Source: CAD feature listing. Evaluate the final solid. Frame: model axes, mm. A direction names the side the tool comes from. Coordinates: 2 decimals unless noted, no trailing zeros. Write each loop counter-clockwise with the first axis right and the second up, starting at its lowest first coordinate (ties: lowest second). Pieces come first, ordered by that corner, then holes. Notation, with made-up numbers: (88.25, -1.5) -> (112.25, -1.5) arc R35 cw to (112.25, 30.5) -> close; hole circle Ø11 at (-20.75, -37.5). An arc over 180 degrees is marked (long way). Write item = value, one per line.
from build123d import *

# Parameters (mm, degrees)
SKETCH1_R             = 3
BOSS_EXTRUDE1_DEPTH   = 2
SKETCH1_R_2           = 1.575
SKETCH1_R_3           = 4.75
BOSS_EXTRUDE1_2_DEPTH = 2
BOSS_EXTRUDE2_DEPTH   = 5.2
FILLET1_R             = 1


with BuildPart() as part:
    # Sketch1 → Boss-Extrude1 (new body)
    with BuildSketch(Plane(origin=(0, 0, 0), x_dir=(1, 0, 0), z_dir=(0, 1, 0))):
        with Locations(Location((0, 0, 0), (0, 0, 270))):
            Circle(SKETCH1_R)
    extrude(amount=BOSS_EXTRUDE1_DEPTH)



with BuildPart() as body_2:
    # Sketch1 → Boss-Extrude1 2 (new body)
    with BuildSketch(Plane(origin=(0, 0, 0), x_dir=(1, 0, 0), z_dir=(0, 1, 0))):
        with BuildLine():
            Line((-2.785823381, 7.172375213), (-8.27733707, 15.397108965))
            Line((-8.27733707, 15.397108965), (-15.361972878, 8.339635234))
            Line((-15.361972878, 8.339635234), (-7.163433576, 2.808735927))
            ThreePointArc((-7.163433576, 2.808735927), (-7.694389311, 0.01229774), (-7.172375213, -2.785823381))
            Line((-7.172375213, -2.785823381), (-15.397108965, -8.27733707))
            Line((-15.397108965, -8.27733707), (-8.339635234, -15.361972878))
            Line((-8.339635234, -15.361972878), (-2.808735927, -7.163433576))
            ThreePointArc((-2.808735927, -7.163433576), (-0.01229774, -7.694389311), (2.785823381, -7.172375213))
            Line((2.785823381, -7.172375213), (8.27733707, -15.397108965))
            Line((8.27733707, -15.397108965), (15.361972878, -8.339635234))
            Line((15.361972878, -8.339635234), (7.163433576, -2.808735927))
            ThreePointArc((7.163433576, -2.808735927), (7.694389311, -0.01229774), (7.172375213, 2.785823381))
            Line((7.172375213, 2.785823381), (15.397108965, 8.27733707))
            Line((15.397108965, 8.27733707), (8.339635234, 15.361972878))
            Line((8.339635234, 15.361972878), (2.808735927, 7.163433576))
            ThreePointArc((2.808735927, 7.163433576), (0.01229774, 7.694389311), (-2.785823381, 7.172375213))
        make_face()
        with Locations(Location((7.61701493, 7.585748715, 0), (0, 0, 270))):
            Circle(SKETCH1_R_2, mode=Mode.SUBTRACT)
        with Locations(Location((0, 0, 0), (0, 0, 270))):
            Circle(SKETCH1_R_3, mode=Mode.SUBTRACT)
        with Locations(Location((-7.61701493, -7.585748715, 0), (0, 0, 270))):
            Circle(SKETCH1_R_2, mode=Mode.SUBTRACT)
        with Locations(Location((-7.585748715, 7.61701493, 0), (0, 0, 270))):
            Circle(SKETCH1_R_2, mode=Mode.SUBTRACT)
        with Locations(Location((7.585748715, -7.61701493, 0), (0, 0, 270))):
            Circle(SKETCH1_R_2, mode=Mode.SUBTRACT)
    extrude(amount=BOSS_EXTRUDE1_2_DEPTH)


with BuildPart() as part_1:
    add(part.part)

    add(body_2.part)  # Boss-Extrude2 merges body 2
    # Sketch1_3 → Boss-Extrude2 (add)
    with BuildSketch(Plane(origin=(0, 0, 0), x_dir=(1, 0, 0), z_dir=(0, 1, 0))):
        with BuildLine():
            Line((-4.622211593, 1.094376528), (-3, 0))
            ThreePointArc((-3, 0), (-2.121320344, 2.121320344), (0, 3))
            Line((0, 3), (-1.084652816, 4.624503029))
            ThreePointArc((-1.084652816, 4.624503029), (-3.355223334, 3.362287373), (-4.622211593, 1.094376528))
        make_face()
        with BuildLine():
            Line((-1.084652816, 4.624503029), (0, 3))
            Line((0, 3), (1.094376528, 4.622211593))
            ThreePointArc((1.094376528, 4.622211593), (0.004995029, 4.749997374), (-1.084652816, 4.624503029))
        make_face()
        with BuildLine():
            Line((1.094376528, 4.622211593), (0, 3))
            ThreePointArc((0, 3), (2.121320344, 2.121320344), (3, 0))
            Line((3, 0), (4.624503029, 1.084652816))
            ThreePointArc((4.624503029, 1.084652816), (4.152794791, 2.305817735), (3.36565776, 3.351842455))
            ThreePointArc((3.36565776, 3.351842455), (2.318714277, 4.145607808), (1.094376528, 4.622211593))
        make_face()
        with BuildLine():
            Line((4.624503029, 1.084652816), (3, 0))
            Line((3, 0), (4.622211593, -1.094376528))
            ThreePointArc((4.622211593, -1.094376528), (4.717944736, -0.550906041), (4.75, 0))
            ThreePointArc((4.75, 0), (4.718521452, 0.545944416), (4.624503029, 1.084652816))
        make_face()
        with BuildLine():
            ThreePointArc((3, 0), (2.121320344, -2.121320344), (0, -3))
            Line((0, -3), (1.084652816, -4.624503029))
            ThreePointArc((1.084652816, -4.624503029), (3.355223334, -3.362287373), (4.622211593, -1.094376528))
            Line((4.622211593, -1.094376528), (3, 0))
        make_face()
        with BuildLine():
            Line((1.084652816, -4.624503029), (0, -3))
            Line((0, -3), (-1.094376528, -4.622211593))
            ThreePointArc((-1.094376528, -4.622211593), (-0.004995029, -4.749997374), (1.084652816, -4.624503029))
        make_face()
        with BuildLine():
            ThreePointArc((0, -3), (-2.121320344, -2.121320344), (-3, 0))
            Line((-3, 0), (-4.624503029, -1.084652816))
            ThreePointArc((-4.624503029, -1.084652816), (-3.362287373, -3.355223334), (-1.094376528, -4.622211593))
            Line((-1.094376528, -4.622211593), (0, -3))
        make_face()
        with BuildLine():
            Line((-4.624503029, -1.084652816), (-3, 0))
            Line((-3, 0), (-4.622211593, 1.094376528))
            ThreePointArc((-4.622211593, 1.094376528), (-4.749997374, 0.004995029), (-4.624503029, -1.084652816))
        make_face()
    extrude(amount=BOSS_EXTRUDE2_DEPTH)

    # Fillet1
    fillet1_edges = [part_1.edges().sort_by_distance(p)[0] for p in [
        (-8.339635234, 1, 15.361972878),
        (-15.397108965, 1, 8.27733707),
        (-15.361972878, 1, -8.339635234),
        (-8.27733707, 1, -15.397108965),
        (8.339635234, 1, -15.361972878),
        (15.397108965, 1, -8.27733707),
        (15.361972878, 1, 8.339635234),
        (8.27733707, 1, 15.397108965),
    ]]
    fillet(fillet1_edges, radius=FILLET1_R)


solid = part_1.part
1) Cut plane B-B, the plane z = -11.25. Output: boundary loops of the cut face in (x, y).
Answer block:
outline = (-12.44, 0) -> (-5.51, 0) -> (-5.51, 2) -> (-12.44, 2) -> close; (5.57, 0) -> (12.44, 0) -> (12.44, 2) -> (5.57, 2) -> close
2) Cut plane A-A, the plane y = 3.9. Output: boundary loops of the cut face in (x, z), and give its area (3 significant figures).
Answer block:
outline = circle Ø9.5 at (0, 0); hole circle Ø6 at (0, 0)
area = 42.6 mm2
3) Cut plane D-D, the plane z = -0.5. Output: boundary loops of the cut face in (x, y), and give its area (3 significant figures).
Answer block:
outline = (-7.68, 0) -> (7.68, 0) -> (7.68, 2) -> (4.72, 2) -> (4.72, 5.2) -> (2.96, 5.2) -> (2.96, 2) -> (-2.96, 2) -> (-2.96, 5.2) -> (-4.72, 5.2) -> (-4.72, 2) -> (-7.68, 2) -> close
area = 42.0 mm2
4) First-contact query: pin 1 Ø1.8 at (x, z) = (0, 0) entering from +Y; pin 2 Ø3 at (x, z) = (7.62, -7.59) entering from -Y; pin 3 Ø3 at (y, z) = (2.5, -11) entering from +X. Flat tips, straight axial feed; report the tip coordinate or a pass-through.
Answer block:
pin_1 = 2
pin_2 = through
pin_3 = 14.09
5) Reachability of faces 1 (the flat face through (-5.16, 0.99, -10.73)), 2 (the flat face through (-11.78, 0.99, -11.91)), 3 (the flat face through (-5.27, 0.99, 10.81)), 4 (the flat face through (10.81, 0.99, 5.27)), 5 (the flat face through (-10.81, 0.99, -5.27)) from +Z, -Z, +X, -X, +Y, -Y: full face, straight path, thin tool, end or side. Return the list, or none.
Answer block:
face_1 = -Z, +Y, -Y
face_2 = -Z, -X, +Y, -Y
face_3 = +Z, +Y, -Y
face_4 = +X, +Y, -Y
face_5 = -X, +Y, -Y
6) Cut plane C-C, the plane x = 10. Output: boundary loops of the cut face in (y, z).
Answer block:
outline = (0, -13.7) -> (2, -13.7) -> (2, -4.67) -> (0, -4.67) -> close; (0, 4.72) -> (2, 4.72) -> (2, 13.68) -> (0, 13.68) -> close
7) Material intervals for probe 1 along Y at (x, z) = (1.5, 1.5); probe 2 along Z at (x, y) = (10.25, 1.6); probe 3 along Z at (x, y) = (9, 0.75), sorted ascending. Write a range as [from, to].
Answer block:
probe_1 = [0, 2]
probe_2 = [-13.44, -4.84], [4.89, 13.43]
probe_3 = [-14.65, -8.34], [-6.83, -4.01], [4.05, 6.92], [8.31, 14.65]
